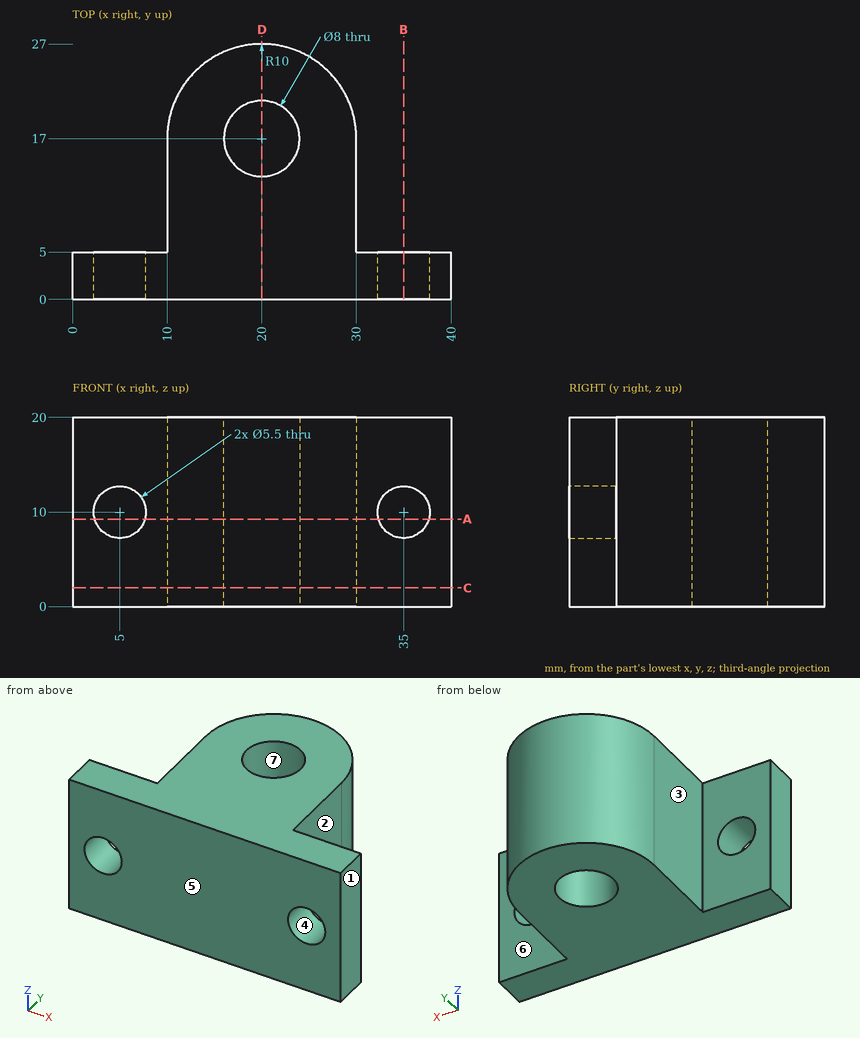
Answer from the drawing. Dimensions are ordinates in mm from the lowest x, y and z of the part. A direction names the side the tool comes from. Coordinates: 2 decimals unless noted, no trailing zeros. Loops run counter-clockwise (first coordinate to the right, second up) from the corner with the lowest first, then second, coordinate; pieces in that order, holes last. Notation, with made-up numbers: (-33, -0.75) -> (4, -0.75) arc R20 cw to (4, 28.25) -> close; hole circle Ø6 at (63, 42). An arc over 180 degrees is marked (long way). Answer as CSV lines item,"result".
Q1. For a pull along Y with two mould halves and no side action, classify the marked faces 4, 5, 6 and 7 as +Y half, -Y half, draft (parallel to the pull), parting line (faces both ways), or undercut.
Findings:
face 4,"draft"
face 5,"-Y half"
face 6,"+Y half"
face 7,"undercut"
Q2. The part is cut by section B-B on x = 35. Write down the section's boundary in (y, z), and give its area (3 significant figures).
Findings:
outline,"(0, 0) -> (5, 0) -> (5, 7.25) -> (0, 7.25) -> close; (0, 12.75) -> (5, 12.75) -> (5, 20) -> (0, 20) -> close"
area,"72.5 mm²"
Q3. Find the intervals of material crossed by probe 1 along X at (y, z) = (2.7, 10); probe 2 along Y at (x, z) = (20, 10); probe 3 along X at (y, z) = (7, 4.5), in increasing order.
Findings:
probe 1,"x = 0 to 2.25, 7.75 to 32.25, 37.75 to 40"
probe 2,"y = 0 to 13, 21 to 27"
probe 3,"x = 10 to 30"
Q4. The part is cut by section C-C on z = 2. Write down the section's boundary in (x, y), and give its area (3 significant figures).
Findings:
outline,"(0, 0) -> (40, 0) -> (40, 5) -> (30, 5) -> (30, 17) arc R10 ccw to (10, 17) -> (10, 5) -> (0, 5) -> close; hole circle Ø8 at (20, 17)"
area,"547 mm²"
Q5. The part is cut by section D-D on x = 20. Write down the section's boundary in (y, z), and give its area (3 significant figures).
Findings:
outline,"(0, 0) -> (13, 0) -> (13, 20) -> (0, 20) -> close; (21, 0) -> (27, 0) -> (27, 20) -> (21, 20) -> close"
area,"380 mm²"
Q6. Each of these flat-tipped pins is pushed along its axis until it touches: pin 1 (7 mm diameter, centred on x = 20, y = 17, fed in from -Z); pin 2 (12 mm diameter, centred on y = 24, z = 3, fed in from +X); pin 3 (6 mm diameter, centred on y = 17.5, z = 13.5, fed in from +X); pin 4 (3 mm diameter, centred on x = 32.5, z = 10.5, fed in from +Y). Where does it stop, or does it pass through?
Findings:
pin 1,"passes through"
pin 2,"stops at x = 29.95"
pin 3,"stops at x = 30"
pin 4,"stops at y = 5"
Q7. A tool of negligible diameter and unlimited length cuts with its end or side. For the marked faces 1, 2 and 3, from which of +Z, -Z, +X, -X, +Y, -Y can it reach the whole face along a straight path? Write none if from no direction.
Findings:
face 1,"+Z, -Z, +X, +Y, -Y"
face 2,"+Z, -Z, +X, +Y"
face 3,"+Z, -Z, -X, +Y"
Q8. The part is cut by section A-A on z = 9.25. Write down the section's boundary in (x, y), and give its area (3 significant figures).
Findings:
outline,"(0, 0) -> (2.35, 0) -> (2.35, 5) -> (0, 5) -> close; (7.65, 0) -> (32.35, 0) -> (32.35, 5) -> (30, 5) -> (30, 17) arc R10 ccw to (10, 17) -> (10, 5) -> (7.65, 5) -> close; (37.65, 0) -> (40, 0) -> (40, 5) -> (37.65, 5) -> close; hole circle Ø8 at (20, 17)"
area,"494 mm²"
